from build123d import *

# Parameters (mm, degrees)
SKETCH1_R           = 13
SKETCH1_R_2         = 10
BOSS_EXTRUDE1_DEPTH = 65
CHAMFER1_SIZE       = 0.5


with BuildPart() as part:
    # Sketch1 → Boss-Extrude1 (new body)
    with BuildSketch(Plane(origin=(0, 0, 0), x_dir=(1, 0, 0), z_dir=(0, 1, 0))):
        with Locations(Location((0, 0, 0), (0, 0, 270))):
            Circle(SKETCH1_R)
        with Locations(Location((0, 0, 0), (0, 0, 270))):
            Circle(SKETCH1_R_2, mode=Mode.SUBTRACT)
    extrude(amount=BOSS_EXTRUDE1_DEPTH)

    # Chamfer1
    chamfer1_edges = [part.edges().sort_by_distance(p)[0] for p in [
        (0, 0, -10),
        (0, 65, -10),
    ]]
    chamfer(chamfer1_edges, length=CHAMFER1_SIZE)

    # Sketch5 → Cut-Revolve4 (revolve, cut)
    with BuildSketch(Plane.XY, mode=Mode.PRIVATE) as cut_revolve4_sk:
        Polygon((-13, 60.948970234), (-12, 60.585), (-9, 60.585), (-9, 60), (-13, 60), align=None)
    revolve(cut_revolve4_sk.sketch.rotate(Axis((-13, 60, 0), (1, 0, 0)), 90), axis=Axis((-13, 60, 0), (1, 0, 0)), mode=Mode.SUBTRACT)


solid = part.part
Verification items for the finished model (mm, model axes). A direction names the side the tool comes from. Coordinates: 2 decimals unless noted, no trailing zeros. Order: outer loops, then holes, each group sorted by start corner. A loop starts at its lowest first (then second) coordinate and runs counter-clockwise, first axis right, second up.
1. Sectioned sample at A-A, the plane x = 0. Record the cut outline in (y, z).
Results found:
outline: (0, -13) - (65, -13) - (65, -10.5) - (64.5, -10) - (0.5, -10) - (0, -10.5) - close; (0, 10.5) - (0.5, 10) - (64.5, 10) - (65, 10.5) - (65, 13) - (0, 13) - close
2. Release check for a two-part mould opening along Z. For faces 1 (the face through (-7.91, 32.045, -10.316)), 2 (the face through (6, 0, -9)), 3 (the face through (-12.271, 60.606, 0.315)) record: +Z half, -Z half, draft (parallel to the pull), parting line (faces both ways), or undercut.
Results found:
face 1: parting line
face 2: draft
face 3: undercut
3. Set-up check for faces 4 (the face through (6, 65, -9)), 5 (the face through (-10.98, 60.57, -0.13)): record each of +Z, -Z, +X, -X, +Y, -Y from which the full face is reachable in a straight line by a thin tool's end or side.
Results found:
face 4: +Z, -Z, +X, -X, +Y
face 5: -X
4. Scan lines: line 1 (Z direction, x = -0.5, y = 9); line 2 (X direction, y = 17.5, z = 0); line 3 (Y direction, x = -11.15, z = 0) (3 decimals). Record each from-to range of solid material in increasing order.
Results found:
line 1: z = -12.99 to -9.99, 9.99 to 12.99
line 2: x = -13 to -10, 10 to 13
line 3: y = 0 to 59.415, 60.585 to 65
5. Go/stop test with flat-tipped pins: pin 1 Ø6 at (x, y) = (-8, 56) entering from -Z; pin 2 Ø2 at (y, z) = (19, -5.5) entering from +X; pin 3 Ø0.7 at (y, z) = (60, 0) entering from -X. Record where each tip stops, or that it passes through.
Results found:
pin 1: stops at z = -12
pin 2: stops at x = 12.2
pin 3: stops at x = 9.99
6. Sectioned sample at B-B, the plane y = 29.5. Record the cut outline in (x, z), and give its area (3 significant figures).
Results found:
outline: circle Ø26 at (0, 0); hole circle Ø20 at (0, 0)
area: 217 mm2
